Input: part model. Units: mm. Frame: model coordinates. Face numbers are marked on the shaded views. A direction names the side the tool comes from. Round coordinates to 2 decimals unless told otherwise and drop trailing zeros. Loops run counter-clockwise (first coordinate to the right, second up) from the corner with the lowest first, then second, coordinate; pieces in that order, holes last.
1) Section C-C, the plane z = 2.25. Return loops of the section in (x, y).
2) Ray query, line 1 along X through (y, z) = (0.5, -3); line 2 along Y through (x, z) = (1, 3.25); line 3 along X through (y, z) = (5.5, -3.5). Return the intervals inside material, ascending.
3) Access query for the marked faces 1 and 2. Directions: +Z, -Z, +X, -X, +Y, -Y. A direction counts if a zero-diameter tool reaches every point of the face in a straight line with its end or side. Return the directions, or none.
4) Section A-A, the plane x = 0. Return loops of the section in (y, z).
5) Draft query along X for the marked faces 3, 4 and 5. Return one class per face: pulls with the +X half, pulls with the -X half, needs draft (parallel to the pull), parting line crosses it, or undercut.
6) Section D-D, the plane y = 13. Return loops of the section in (x, z).
7) First-contact query: pin 1 (1 mm diameter, centred on x = -5, z = -4, fed in from -Y); pin 2 (2 mm diameter, centred on x = -4.5, z = -2, fed in from -Y); pin 3 (3.5 mm diameter, centred on y = -4, z = -1.5, fed in from -X). Flat tips, straight axial feed; report the tip coordinate or a pass-through.
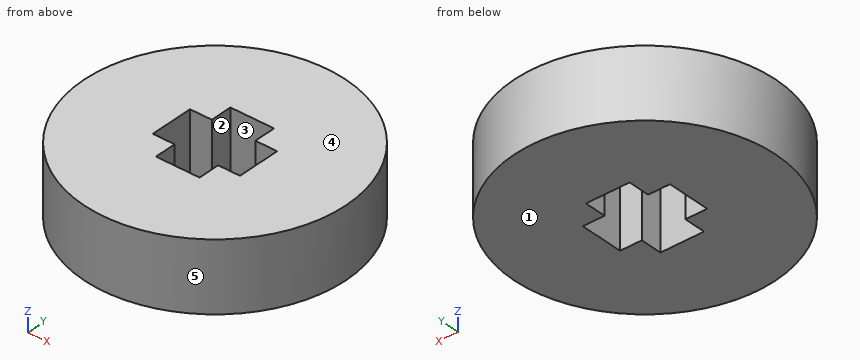
Autodesk Inventor part; units mm, degrees
ref_plane "YZ Plane" through (0, 0, 0) normal (1, 0, 0) x (0, 1, 0)
ref_plane "XZ Plane" through (0, 0, 0) normal (0, 1, 0) x (-1, 0, 0)
ref_plane "XY Plane" through (0, 0, 0) normal (0, 0, 1) x (1, 0, 0)
sketch "Sketch1" plane through (0, 0, 0) normal (0, 0, 1) x (1, 0, 0)
  circle A0 centre (0, 0) radius 18
  dimension "d0" = 36
extrude "Extrusion1" add sketch "Sketch1" along normal mid plane 9.5
sketch "Sketch2" plane through (0, 0, -4.75) normal (0, 0, -1) x (-1, 0, 0)
  line L0 (0, 0) -> (0, 6)
  line L1 (0, 6) -> (3, 6)
  line L2 (3, 6) -> (3, 3)
  line L3 (3, 3) -> (6, 3)
  line L4 (6, 3) -> (6, -3)
  line L5 (6, -3) -> (3, -3)
  line L6 (3, -3) -> (3, -6)
  line L7 (3, -6) -> (-3, -6)
  line L8 (-3, -6) -> (-3, -3)
  line L9 (-3, -3) -> (-6, -3)
  line L10 (-6, -3) -> (-6, 3)
  line L11 (-6, 3) -> (-3, 3)
  line L12 (-3, 3) -> (-3, 6)
  line L13 (-3, 6) -> (0, 6)
  dimension "d46" = 6
  dimension "d47" = 3
  dimension "d48" = 3
  dimension "d49" = 3
  dimension "d50" = 6
  dimension "d51" = 3
  dimension "d52" = 3
  dimension "d53" = 6
  dimension "d55" = 3
  dimension "d56" = 3
  dimension "d57" = 6
  dimension "d59" = 3
  dimension "d60" = 3
extrude "Extrusion2" cut sketch "Sketch2" against normal blind 11
properties part number "OmniShaft"
Final values:
1. outline: circle Ø36 at (0, 0); hole (-6, -3) - (-3, -3) - (-3, -6) - (3, -6) - (3, -3) - (6, -3) - (6, 3) - (3, 3) - (3, 6) - (-3, 6) - (-3, 3) - (-6, 3) - close
2. line 1: x = -17.99 to -6, 6 to 17.99
2. line 2: y = -17.97 to -6, 6 to 17.97
2. line 3: x = -17.14 to -3, 3 to 17.14
3. face 1: -Z, +X, -X, +Y, -Y
3. face 2: +Z, -Z
4. outline: (-18, -4.75) - (-6, -4.75) - (-6, 4.75) - (-18, 4.75) - close; (6, -4.75) - (18, -4.75) - (18, 4.75) - (6, 4.75) - close
5. face 3: undercut
5. face 4: needs draft
5. face 5: parting line crosses it
6. outline: (-12.45, -4.75) - (12.45, -4.75) - (12.45, 4.75) - (-12.45, 4.75) - close
7. pin 1: stops at y = -17.43
7. pin 2: stops at y = -17.66
7. pin 3: stops at x = -17.86
